Build history of the part. All positions in model axes, mm. A direction names the side the tool comes from. Give positions to 0.01 mm unless a question says otherwise; leave off trailing zeros. Loops run counter-clockwise (first coordinate to the right, second up) from the corner with the lowest first, then second, coordinate; pieces in that order, holes last. Notation, with made-up numbers: M -10,22.25 L 31,22.25 A12 cw 31,26.25 Z; hole C -9.75,25 d9. An arc over 180 degrees is marked long. Answer in a Markdown table with one row per item. Add a question column.
```python
from build123d import *

# Parameters (mm, degrees)
SKETCH1_W           = 26
SKETCH1_H           = 17
BOSS_EXTRUDE1_DEPTH = 4
SKETCH2_W           = 3
SKETCH2_H           = 17
BOSS_EXTRUDE2_DEPTH = 35
SKETCH3_R           = 2.75
CUT_EXTRUDE1_DEPTH  = 45.421278685
FILLET1_R           = 3
FILLET2_R           = 5
SKETCH5_R           = 7
BOSS_EXTRUDE3_DEPTH = 2
CUT_EXTRUDE3_REACH  = 43.979
SKETCH7_R           = 2.25
CUT_EXTRUDE4_DEPTH  = 4
CHAMFER1_SIZE       = 2


with BuildPart() as part:
    # Sketch1 → Boss-Extrude1 (new body)
    with BuildSketch(Plane(origin=(0, 0, 0), x_dir=(0, 0, -1), z_dir=(1, 0, 0))):
        Rectangle(SKETCH1_W, SKETCH1_H)
    extrude(amount=BOSS_EXTRUDE1_DEPTH)

    # Sketch2 → Boss-Extrude2 (add)
    with BuildSketch(Plane.ZY):
        with Locations((-11.5, 0)):
            Rectangle(SKETCH2_W, SKETCH2_H)
        with Locations((11.5, 0)):
            Rectangle(SKETCH2_W, SKETCH2_H)
    extrude(amount=BOSS_EXTRUDE2_DEPTH)

    # Sketch3 → Cut-Extrude1 (cut, through all)
    with BuildSketch(Plane.XY.offset(13)):
        with Locations((-29.5, 0)):
            Circle(SKETCH3_R)
    extrude(amount=-CUT_EXTRUDE1_DEPTH, mode=Mode.SUBTRACT)

    # Fillet1
    fillet1_edges = [part.edges().sort_by_distance(p)[0] for p in [
        (4, 0, 13),
        (0, 0, -10),
        (0, 0, 10),
        (4, 0, -13),
    ]]
    fillet(fillet1_edges, radius=FILLET1_R)

    # Fillet2
    fillet2_edges = [part.edges().sort_by_distance(p)[0] for p in [
        (-35, -8.5, -11.5),
        (-35, 8.5, -11.5),
        (-35, 8.5, 11.5),
        (-35, -8.5, 11.5),
    ]]
    fillet(fillet2_edges, radius=FILLET2_R)

    # Sketch5 → Boss-Extrude3 (add)
    with BuildSketch(Plane.ZY):
        Circle(SKETCH5_R)
    extrude(amount=BOSS_EXTRUDE3_DEPTH)

    # Sketch7 → Cut-Extrude3 (cut, up to next)
    with BuildSketch(Plane(origin=(4, 0, 0), x_dir=(0, 0, -1), z_dir=(1, 0, 0)), mode=Mode.PRIVATE) as cut_extrude3_sk1:
        Circle(SKETCH7_R)
    cut_extrude3_tool1 = extrude(cut_extrude3_sk1.sketch, amount=-CUT_EXTRUDE3_REACH, mode=Mode.PRIVATE) & part.part
    add(cut_extrude3_tool1.solids().sort_by_distance((4, 0, 0))[0], mode=Mode.SUBTRACT)

    # Sketch8 → Cut-Extrude4 (cut)
    with BuildSketch(Plane.ZY.offset(2)):
        Polygon((0, 4.330127019), (-3.75, 2.165063509), (-3.75, -2.165063509), (0, -4.330127019), (3.75, -2.165063509), (3.75, 2.165063509), align=None)
    extrude(amount=-CUT_EXTRUDE4_DEPTH, mode=Mode.SUBTRACT)

    # Chamfer1
    # the kernel refuses this chamfer: 2 mm, written as the material it adds along each edge
    with BuildSketch(Plane(origin=(0, 0, 0), x_dir=(0, 0, 1), z_dir=(0, -1, 0))) as chamfer1_piece_1_section:
        Polygon((7 + CHAMFER1_SIZE, 0), (7, CHAMFER1_SIZE), (7, 0), align=None)
    chamfer1_piece_1 = revolve(axis=Axis((0, 0, 0), (-1, 0, 0)), revolution_arc=180, mode=Mode.PRIVATE)
    chamfer1_piece_1 = split(chamfer1_piece_1, bisect_by=Plane(origin=(-0.945270908, 8.5, 0), z_dir=(0, -1, 0)), keep=Keep.TOP, mode=Mode.PRIVATE)
    chamfer1_piece_1 = split(chamfer1_piece_1, bisect_by=Plane(origin=(-2, 8.001839451, 0), z_dir=(1, 0, 0)), keep=Keep.TOP, mode=Mode.PRIVATE)
    add(chamfer1_piece_1)
    with BuildSketch(Plane(origin=(0, 0, 0), x_dir=(0, 0, -1), z_dir=(0, 1, 0))) as chamfer1_piece_2_section:
        Polygon((7 + CHAMFER1_SIZE, 0), (7, CHAMFER1_SIZE), (7, 0), align=None)
    chamfer1_piece_2 = revolve(axis=Axis((0, 0, 0), (-1, 0, 0)), revolution_arc=180, mode=Mode.PRIVATE)
    chamfer1_piece_2 = split(chamfer1_piece_2, bisect_by=Plane(origin=(-0.945270905, -8.5, 0), z_dir=(0, 1, 0)), keep=Keep.TOP, mode=Mode.PRIVATE)
    chamfer1_piece_2 = split(chamfer1_piece_2, bisect_by=Plane(origin=(-2, -8.001839447, 0), z_dir=(1, 0, 0)), keep=Keep.TOP, mode=Mode.PRIVATE)
    add(chamfer1_piece_2)


solid = part.part
```
(1) Pull direction Y, two halves, no side cores. Call faces 4 (the flat face through (2, -2, -2)), 5 (the flat face through (-19, 0, -10)), 6 (the flat face through (0, -8.5, 1)): +Y half, -Y half, draft (parallel to the pull), parting line (faces both ways), or undercut.
(2) Slice it at B-B, the plane y = 0. State how many separate pieces and enclosed holes the cut face has, then the cut area to 3 significant figures.
(3) Slice it at C-C, the plane x = -29.5. Give the cut face in (y, z), then the cut area to 3 significant figures.
(4) Pin check, flat tips, straight feed: pin 1 (3 mm diameter, centred on y = -7, z = -5, fed in from -X); pin 2 (5 mm diameter, centred on y = 2, z = -3.5, fed in from -X); pin 3 (4 mm diameter, centred on y = -1, z = -1.5, fed in from -X). Stop position of each tip, or through.
(5) Slice it at D-D, the plane z = 11. Give the cut face in (x, y), then the cut area to 3 significant figures.
(6) Slice it at A-A, the plane x = -5. Give the cut face in (y, z).
(7) Wall check: line 1 (Y direction, x = -29.5, z = -11.2); line 2 (Z direction, x = -18.5, y = -0.5); line 3 (Y direction, x = 2.9, z = 0). Give the ranges that are in metal, low to high.
(8) Tool access for faces 1 (the flat face through (-0.028, 3.232, 1.901)), 2 (the flat face through (0, -8, 6)), 3 (the cylindrical face through (3.14, 0.12, 12.1)): list every direction of +Z, -Z, +X, -X, +Y, -Y with a clear straight run to the whole face (end or side of a thin tool).
Solution:
| question | item | result |
|---|---|---|
| 1 | face 4 | undercut |
| 1 | face 5 | draft |
| 1 | face 6 | -Y half |
| 2 | separate pieces | 4 |
| 2 | enclosed holes | 0 |
| 2 | area | 273 mm^2 |
| 3 | outline | M -8.5,-13 L -2.75,-13 L -2.75,-10 L -8.5,-10 Z; M -8.5,10 L -2.75,10 L -2.75,13 L -8.5,13 Z; M 2.75,-13 L 8.5,-13 L 8.5,-10 L 2.75,-10 Z; M 2.75,10 L 8.5,10 L 8.5,13 L 2.75,13 Z |
| 3 | area | 69.0 mm^2 |
| 4 | pin 1 | x = -1.9 |
| 4 | pin 2 | x = -2 |
| 4 | pin 3 | x = 2 |
| 5 | outline | M -35,-3.5 A5 ccw -30,-8.5 L 3.83,-8.5 L 3.83,8.5 L -30,8.5 A5 ccw -35,3.5 Z; hole C -29.5,0 d5.5 |
| 5 | area | 626 mm^2 |
| 6 | outline | M -8.5,-13 L 8.5,-13 L 8.5,-10 L -8.5,-10 Z; M -8.5,10 L 8.5,10 L 8.5,13 L -8.5,13 Z |
| 7 | line 1 | -8.5 to -2.75, 2.75 to 8.5 |
| 7 | line 2 | -13 to -10, 10 to 13 |
| 7 | line 3 | -8.5 to -2.25, 2.25 to 8.5 |
| 8 | face 1 | -X |
| 8 | face 2 | -X, -Y |
| 8 | face 3 | +Z, +X, +Y, -Y |
